from build123d import *

# Parameters (mm, degrees)
BOSS_EXTRUDE1_DEPTH = 7.62
SKETCH4_R           = 10.16
BOSS_EXTRUDE2_DEPTH = 12.7
SKETCH5_R           = 11.43
SKETCH5_R_2         = 10.16
EXTRUDE_THIN1_DEPTH = 7.62
CHAMFER2_SIZE       = 0.254
CHAMFER2_SIZE2      = 0.146646968
CUT_SWEEP4_PITCH    = 2.54
CUT_SWEEP4_TO       = 7.62
SKETCH10_R          = 26.67
BOSS_EXTRUDE3_DEPTH = 279.4
SKETCH11_R          = 1.27
BOSS_EXTRUDE4_DEPTH = 6.35
SKETCH12_R          = 1.27
BOSS_EXTRUDE5_DEPTH = 6.35
SKETCH13_R          = 1.27
BOSS_EXTRUDE6_DEPTH = 6.35
SKETCH14_R          = 1.27
BOSS_EXTRUDE7_DEPTH = 6.35
SKETCH16_R          = 1.016
BOSS_EXTRUDE8_DEPTH = 6.35
SKETCH17_R          = 26.67
BOSS_EXTRUDE9_DEPTH = 127


with BuildPart() as part:
    # Sketch3 → Boss-Extrude1 (new body)
    with BuildSketch(Plane(origin=(0, 0, 0), x_dir=(0, 0, -1), z_dir=(1, 0, 0))):
        Polygon((14.662463333, 0.255934249), (7.109586105, 12.826032853), (-7.552877228, 12.570098604), (-14.662463333, -0.255934249), (-7.109586105, -12.826032853), (7.552877228, -12.570098604), align=None)
    extrude(amount=BOSS_EXTRUDE1_DEPTH)

    # Sketch4 → Boss-Extrude2 (add)
    with BuildSketch(Plane(origin=(7.62, 0, 0), x_dir=(0, 0, -1), z_dir=(1, 0, 0))):
        Circle(SKETCH4_R)
    extrude(amount=BOSS_EXTRUDE2_DEPTH)

    # Sketch5 → Extrude-Thin1 (add)
    with BuildSketch(Plane(origin=(7.62, 0, 0), x_dir=(0, 0, -1), z_dir=(1, 0, 0))):
        Circle(SKETCH5_R)
        Circle(SKETCH5_R_2, mode=Mode.SUBTRACT)
    extrude(amount=EXTRUDE_THIN1_DEPTH)

    # Chamfer2
    chamfer2_edges = [part.edges().sort_by_distance(p)[0] for p in [
        (15.24, 0, 11.43),
    ]]
    chamfer2_side = [part.faces().sort_by_distance(p)[0] for p in [
        (11.43, 0, 11.43),
    ]]
    chamfer(chamfer2_edges, length=CHAMFER2_SIZE, length2=CHAMFER2_SIZE2, reference=chamfer2_side[0])

    # Cut-Sweep4: arcs per turn and ends read off the stored shape
    # Cut-Sweep4: the profile of Sketch9 screwed along a right-hand helix through 3.6 turns, 10 arcs to a turn; built about Z, then put on its axis
    cut_sweep4_z = Axis((0, 0, 0), (0, 0, 1))
    cut_sweep4_corners = [(10.414, 0, 0), (11.938, 0, -0.87988181), (11.938, 0, 0.87988181)]
    with BuildLine(mode=Mode.PRIVATE) as cut_sweep4_profile:
        Line(cut_sweep4_corners[0], cut_sweep4_corners[1])
        Line(cut_sweep4_corners[1], cut_sweep4_corners[2])
        Line(cut_sweep4_corners[2], cut_sweep4_corners[0])
    cut_sweep4_cap = Face(cut_sweep4_profile.wire())
    cut_sweep4_turn_angles = [0, 18, 36, 54, 72, 90, 108, 126, 144, 162, 180, 198, 216, 234, 252, 270, 288, 306, 324, 342, 360]
    cut_sweep4_turn_weights = [1, 0.9510565162951535, 1, 0.9510565162951535, 1, 0.9510565162951535, 1, 0.9510565162951535, 1, 0.9510565162951535, 1, 0.9510565162951535, 1, 0.9510565162951535, 1, 0.9510565162951535, 1, 0.9510565162951535, 1, 0.9510565162951535, 1]
    cut_sweep4_turn_rails = [Edge.make_bspline([Vector(p[0], p[1], 0).rotate(cut_sweep4_z, cut_sweep4_turn_angles[k]) / cut_sweep4_turn_weights[k] + Vector(0, 0, p[2] + CUT_SWEEP4_PITCH * cut_sweep4_turn_angles[k] / 360) for k in range(21)], [0, 0, 0, 1, 1, 2, 2, 3, 3, 4, 4, 5, 5, 6, 6, 7, 7, 8, 8, 9, 9, 10, 10, 10], 2, cut_sweep4_turn_weights) for p in cut_sweep4_corners]
    cut_sweep4_turn_sides = [Face.make_surface_from_curves(cut_sweep4_turn_rails[p[0]], cut_sweep4_turn_rails[p[1]]) for p in [(0, 1), (1, 2), (2, 0)]]
    cut_sweep4_last_angles = [1080, 1098, 1116, 1134, 1152, 1170, 1188, 1206, 1224, 1242, 1260, 1278, 1296]
    cut_sweep4_last_weights = [1, 0.9510565162951535, 1, 0.9510565162951535, 1, 0.9510565162951535, 1, 0.9510565162951535, 1, 0.9510565162951535, 1, 0.9510565162951535, 1]
    cut_sweep4_last_rails = [Edge.make_bspline([Vector(p[0], p[1], 0).rotate(cut_sweep4_z, cut_sweep4_last_angles[k]) / cut_sweep4_last_weights[k] + Vector(0, 0, p[2] + CUT_SWEEP4_PITCH * cut_sweep4_last_angles[k] / 360) for k in range(13)], [0, 0, 0, 1, 1, 2, 2, 3, 3, 4, 4, 5, 5, 6, 6, 6], 2, cut_sweep4_last_weights) for p in cut_sweep4_corners]
    cut_sweep4_last_sides = [Face.make_surface_from_curves(cut_sweep4_last_rails[p[0]], cut_sweep4_last_rails[p[1]]) for p in [(0, 1), (1, 2), (2, 0)]]
    cut_sweep4 = Plane(origin=(15.24, 0, 0), x_dir=(0, 0, -1), z_dir=(-1, 0, 0)) * split(Solid(Shell([*[p.moved(Location((0, 0, CUT_SWEEP4_PITCH * i))) for i in range(3) for p in cut_sweep4_turn_sides], *cut_sweep4_last_sides, cut_sweep4_cap, cut_sweep4_cap.rotate(cut_sweep4_z, 1296).moved(Location((0, 0, CUT_SWEEP4_PITCH * 1296 / 360)))])), bisect_by=Plane.XY.offset(CUT_SWEEP4_TO), keep=Keep.BOTTOM, mode=Mode.PRIVATE)
    add(cut_sweep4, mode=Mode.SUBTRACT)

    # Sketch10 → Boss-Extrude3 (add)
    with BuildSketch(Plane.ZY):
        Circle(SKETCH10_R)
    extrude(amount=BOSS_EXTRUDE3_DEPTH)

    # Sketch11 → Boss-Extrude4 (add)
    with BuildSketch(Plane(origin=(20.32, 0, 0), x_dir=(0, 0, -1), z_dir=(1, 0, 0))):
        with Locations((-3.048, 3.048)):
            Circle(SKETCH11_R)
    extrude(amount=BOSS_EXTRUDE4_DEPTH)

    # Sketch12 → Boss-Extrude5 (add)
    with BuildSketch(Plane(origin=(20.32, 0, 0), x_dir=(0, 0, -1), z_dir=(1, 0, 0))):
        with Locations((3.048, 3.048)):
            Circle(SKETCH12_R)
    extrude(amount=BOSS_EXTRUDE5_DEPTH)

    # Sketch13 → Boss-Extrude6 (add)
    with BuildSketch(Plane(origin=(20.32, 0, 0), x_dir=(0, 0, -1), z_dir=(1, 0, 0))):
        with Locations((3.048, -3.048)):
            Circle(SKETCH13_R)
    extrude(amount=BOSS_EXTRUDE6_DEPTH)

    # Sketch14 → Boss-Extrude7 (add)
    with BuildSketch(Plane(origin=(20.32, 0, 0), x_dir=(0, 0, -1), z_dir=(1, 0, 0))):
        with Locations((-3.048, -3.048)):
            Circle(SKETCH14_R)
    extrude(amount=BOSS_EXTRUDE7_DEPTH)

    # Sketch16 → Boss-Extrude8 (add)
    with BuildSketch(Plane(origin=(20.32, 0, 0), x_dir=(0, 0, -1), z_dir=(1, 0, 0))):
        with Locations((0, 6.35)):
            Circle(SKETCH16_R)
    extrude(amount=BOSS_EXTRUDE8_DEPTH)

    # Sketch17 → Boss-Extrude9 (add)
    with BuildSketch(Plane(origin=(0, 0, 0), x_dir=(0, 0, -1), z_dir=(1, 0, 0))):
        with Locations(Location((0, 0, 0), (0, 0, 180))):
            Circle(SKETCH17_R)
    extrude(amount=-BOSS_EXTRUDE9_DEPTH)


solid = part.part
Source: CAD feature listing. Evaluate the final solid. Frame: model axes, mm. A direction names the side the tool comes from. Give positions to 0.01 mm unless a question says otherwise; leave off trailing zeros. Write each loop counter-clockwise with the first axis right and the second up, starting at its lowest first coordinate (ties: lowest second). Pieces come first, ordered by that corner, then holes. Notation, with made-up numbers: (43.25, 79) -> (57.25, 79) arc R23 ccw to (57.25, 87) -> close; hole circle Ø1 at (-2, 28). An arc over 180 degrees is marked (long way). Return JSON: item names as keys, results as strings. Group by question number.
1. Section A-A, the plane x = -28. Output: boundary loops of the cut face in (y, z).
2. Pin query (flat end, axial travel): pin 1 Ø22.5 at (y, z) = (-4.5, 0) entering from +X; pin 2 Ø1 at (y, z) = (21, 5.5) entering from +X; pin 3 Ø1.5 at (x, y) = (-150, -14.5) entering from +Z; pin 4 Ø4 at (x, z) = (-171.5, -20) entering from +Y. Return the tip coordinate at first contact, or that it passes through.
3. Material intervals for line 1 (X direction, y = -7.5, z = 8.5); line 2 (X direction, y = 16.5, z = 1.5); line 3 (X direction, y = -3.5, z = 6.5), sorted ascending. Write a range as from..to.
4. Section B-B, the plane z = 17.5. Output: boundary loops of the cut face in (x, y), then the cut area to 3 significant figures.
5. Access query for faces 1 (the face through (20.32, 0, 0)), 2 (the face through (3.76, -6.45, 10.94)), 3 (the face through (3.76, 6.45, -10.94)), 4 (the face through (3.757, 6.247, 11.058)). Directions: +Z, -Z, +X, -X, +Y, -Y. A direction counts if a zero-diameter tool reaches every point of the face in a straight line with its end or side. Return the directions, or none.
Determined:
{
 "1": {"outline": "circle Ø53.34 at (0, 0)"},
 "2": {"pin 1": "stops at x = 26.67", "pin 2": "stops at x = 0", "pin 3": "stops at z = 22.85", "pin 4": "stops at y = 19.68"},
 "3": {"line 1": "x = -279.4..8.65, 9.71..11.19, 12.25..13.73, 14.79..15.15", "line 2": "x = -279.4..0", "line 3": "x = -279.4..20.32"},
 "4": {"outline": "(-279.4, -20.13) -> (0, -20.13) -> (0, 20.13) -> (-279.4, 20.13) -> close", "area": "11,200 mm2"},
 "5": {"face 1": "+X", "face 2": "+Z, +X, -Y", "face 3": "-Z, +X, +Y", "face 4": "+Z, +X, +Y"}
}
